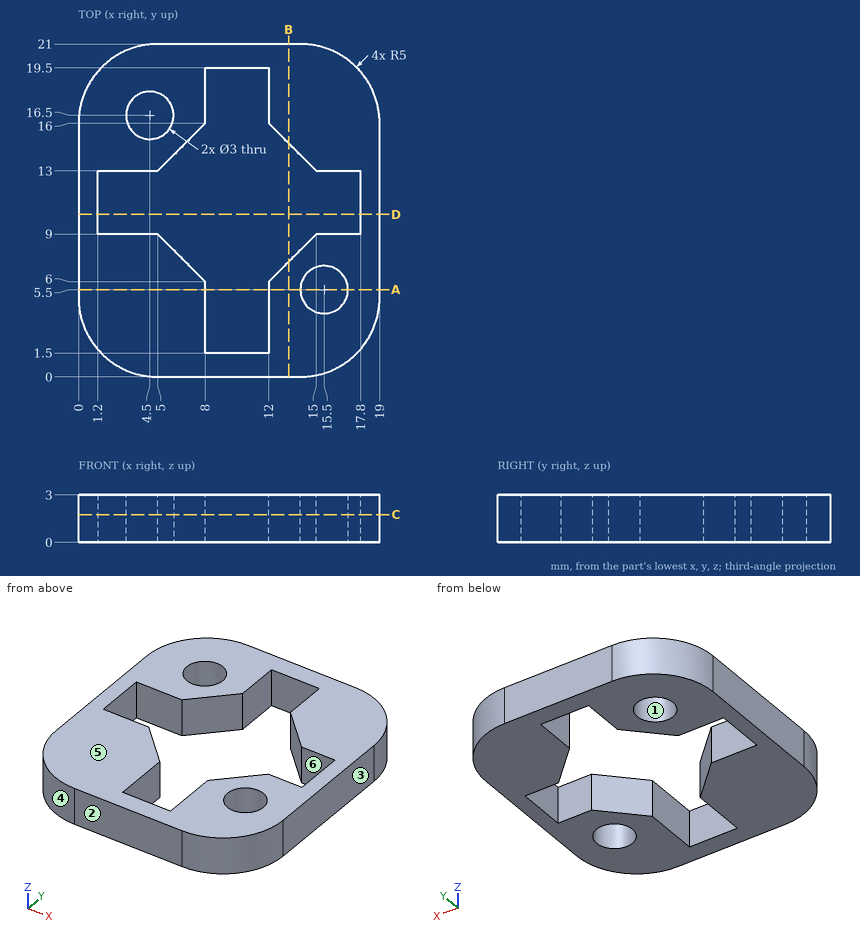
Study the drawing (mm; zero at the part's minimum x, y, z) and answer. A direction names the side the tool comes from. Round coordinates to 2 decimals unless told otherwise and drop trailing zeros. Loops run counter-clockwise (first coordinate to the right, second up) from the corner with the lowest first, then second, coordinate; pieces in that order, holes last. Notation, with made-up numbers: (48, 28.5) -> (86, 28.5) arc R15 ccw to (86, 38.5) -> close; hole circle Ø7 at (-34.75, 84.25). An arc over 180 degrees is marked (long way). Use one line per item in the form item = value.
1. A flat-ended cylindrical pin translates along its axis: pin 1 Ø0.9 at (y, z) = (17, 2) entering from -X. Find the tip coordinate at first contact, or state that the pin passes through.
Answer key:
pin_1 = 0.03
2. The part is cut by section C-C on z = 1.75. Determine the outline of the cut face in (x, y).
Answer key:
outline = (0, 5) arc R5 ccw to (5, 0) -> (14, 0) arc R5 ccw to (19, 5) -> (19, 16) arc R5 ccw to (14, 21) -> (5, 21) arc R5 ccw to (0, 16) -> close; hole (1.2, 9) -> (5, 9) -> (8, 6) -> (8, 1.5) -> (12, 1.5) -> (12, 6) -> (15, 9) -> (17.8, 9) -> (17.8, 13) -> (15, 13) -> (12, 16) -> (12, 19.5) -> (8, 19.5) -> (8, 16) -> (5, 13) -> (1.2, 13) -> close; hole circle Ø3 at (4.5, 16.5); hole circle Ø3 at (15.5, 5.5)
3. The part is cut by section B-B on x = 13.25. Determine the outline of the cut face in (y, z).
Answer key:
outline = (0, 0) -> (7.25, 0) -> (7.25, 3) -> (0, 3) -> close; (14.75, 0) -> (21, 0) -> (21, 3) -> (14.75, 3) -> close
4. For a pull along X with two mould halves and no side action, classify the marked faces 1, 2, 3 and 4 as released by +X, released by -X, zero draft, split by the parting line, or undercut.
Answer key:
face_1 = undercut
face_2 = zero draft
face_3 = released by +X
face_4 = released by -X
5. The part is cut by section A-A on y = 5.5. Determine the outline of the cut face in (x, z), and give its area (3 significant figures).
Answer key:
outline = (0, 0) -> (8, 0) -> (8, 3) -> (0, 3) -> close; (12, 0) -> (14, 0) -> (14, 3) -> (12, 3) -> close; (17, 0) -> (19, 0) -> (19, 3) -> (17, 3) -> close
area = 36.0 mm²
6. The part is cut by section D-D on y = 10.25. Determine the outline of the cut face in (x, z), and give its area (3 significant figures).
Answer key:
outline = (0, 0) -> (1.2, 0) -> (1.2, 3) -> (0, 3) -> close; (17.8, 0) -> (19, 0) -> (19, 3) -> (17.8, 3) -> close
area = 7.20 mm²
7. A tool of negligible diameter and unlimited length cuts with its end or side. For the marked faces 5 and 6, from which of +Z, -Z, +X, -X, +Y, -Y can it reach the whole face along a straight path? Write none if from no direction.
Answer key:
face_5 = +Z, +X, -X, +Y, -Y
face_6 = +Z, -Z
8. Find the intervals of material crossed by probe 1 along Y at (x, z) = (4.5, 1.2); probe 2 along X at (y, z) = (17.25, 2.6); probe 3 along X at (y, z) = (12.5, 2.85), in increasing order. Write a range as [from, to].
Answer key:
probe_1 = [0.03, 9], [13, 15], [18, 20.97]
probe_2 = [0.16, 3.2], [5.8, 8], [12, 18.84]
probe_3 = [0, 1.2], [17.8, 19]
